from build123d import *

# Parameters (mm, degrees)
SKETCH1_W           = 25.4
SKETCH1_H           = 25.4
SKETCH1_W_2         = 22.098
SKETCH1_H_2         = 22.098
BOSS_EXTRUDE1_DEPTH = 365.442999
SKETCH5_W           = 25.4
SKETCH5_H           = 25.4
CUT_EXTRUDE2_DEPTH  = 244.121497904
CUT_EXTRUDE3_DEPTH  = 26.4


with BuildPart() as part:
    # Sketch1 → Boss-Extrude1 (new body)
    with BuildSketch(Plane.XY):
        Rectangle(SKETCH1_W, SKETCH1_H)
        Rectangle(SKETCH1_W_2, SKETCH1_H_2, mode=Mode.SUBTRACT)
    extrude(amount=BOSS_EXTRUDE1_DEPTH)

    # Sketch5 → Cut-Extrude2 (cut, through all)
    with BuildSketch(Plane(origin=(0, 132.21706056, 169.900698991), x_dir=(-1, 0, 0), z_dir=(0, 0.557172611, -0.830396701))):
        Rectangle(SKETCH5_W, SKETCH5_H)
    extrude(amount=-CUT_EXTRUDE2_DEPTH, mode=Mode.SUBTRACT)

    # Sketch6 → Cut-Extrude3 (cut, through all)
    with BuildSketch(Plane.ZY.offset(12.7)):
        Polygon((0, -12.7), (25.987122875, 17.048162291), (0, 20.823213659), align=None)
    extrude(amount=-CUT_EXTRUDE3_DEPTH, mode=Mode.SUBTRACT)


solid = part.part
CAD build for the part. Positions are in the model's coordinates, mm. A direction names the side the tool comes from. Round coordinates to 2 decimals unless told otherwise and drop trailing zeros. Write each loop counter-clockwise with the first axis right and the second up, starting at its lowest first coordinate (ties: lowest second). Pieces come first, ordered by that corner, then holes. Notation, with made-up numbers: M -28.75,-33 L 2.25,-33 A19 cw 2.25,-17 Z; hole C -18,88.25 d10. An arc over 180 degrees is marked long. Use a Markdown table: item, result. Add a question column.
1. Drill centre lines: probe 1 along Y at (x, z) = (-2, 123); probe 2 along Y at (x, z) = (0.5, 16). Where is each one in solid material? Low to high.
2. Flat gauge pins, fed straight in: P1, Ø10, axis at x = -8.5, y = 6, coming from the +Z side; P2, Ø6, axis at x = -10, y = -0.5, coming from the +Z side. Where does each tip first touch, or does it go through?
3. Slice it at C-C on y = 5.75. Give the cut face in (x, z), then the cut area to 3 significant figures.
4. Pull direction Y, two halves, no side cores. Call faces 3 (the face through (12.7, 0, 179)), 4 (the face through (-11.467, -0.178, 10.939)), 5 (the face through (-11.049, 0, 179)): released by +Y, released by -Y, zero draft, split by the parting line, or undercut.
5. Slice it at A-A on z = 183. Give the cut face in (x, y), then the cut area to 3 significant figures.
6. Slice it at B-B on x = -5.5. Give the cut face in (y, z), then the cut area to 3 significant figures.
7. 3-axis set-ups, long thin cutter, end or side, ignore diameter. For faces 1 (the face through (0, -11.049, 179)), 2 (the face through (0, 12.7, 172)): which of +Z, -Z, +X, -X, +Y, -Y reach the whole face in a straight line?
Reply:
| question | item | result |
|---|---|---|
| 1 | probe 1 | y = -12.7 to -11.05, 11.05 to 12.7 |
| 1 | probe 2 | y = -12.7 to -11.05 |
| 2 | P1 | stops at z = 341.63 |
| 2 | P2 | stops at z = 349.09 |
| 3 | outline | M -12.7,16.12 L -11.05,16.12 L -11.05,335.59 L -12.7,335.59 Z; M 11.05,16.12 L 12.7,16.12 L 12.7,335.59 L 11.05,335.59 Z |
| 3 | area | 1,050 mm^2 |
| 4 | face 3 | zero draft |
| 4 | face 4 | released by +Y |
| 4 | face 5 | undercut |
| 5 | outline | M -12.7,-12.7 L 12.7,-12.7 L 12.7,12.7 L -12.7,12.7 Z; hole M -11.05,-11.05 L 11.05,-11.05 L 11.05,11.05 L -11.05,11.05 Z |
| 5 | area | 157 mm^2 |
| 6 | outline | M -12.7,0 L -11.05,1.44 L -11.05,360.63 L -12.7,363.09 Z; M 11.05,20.75 L 12.7,22.19 L 12.7,325.23 L 11.05,327.69 Z |
| 6 | area | 1,100 mm^2 |
| 7 | face 1 | +Z, -Z |
| 7 | face 2 | +Z, -Z, +X, -X, +Y |
